```python
from build123d import *

# Parameters (mm, degrees)
F1_DEPTH  = 10
F2_W      = 5
F2_H      = 20
F3_DEPTH  = 20
F5_DEPTH  = 3
F8_DEPTH  = 12
F9_R      = 5.5
F10_DEPTH = 20
F11_R     = 2.65
F12_DEPTH = 25
F13_R     = 3.15
F14_DEPTH = 25
F16_DEPTH = 20
F18_DEPTH = 25


with BuildPart() as f1:
    # F0 (on Front) → F1 (new body, symmetric)
    with BuildSketch(Plane.XZ):
        Polygon((-10, 20), (-10, -20), (10, -10), (10, 10), align=None)
    extrude(amount=F1_DEPTH, both=True)

    # F2 (on face) → F3 (join, through all)
    with BuildSketch(Plane.XZ.offset(10)):
        with Locations((12.5, 0)):
            Rectangle(F2_W, F2_H)
    extrude(amount=-F3_DEPTH)

    # F4 (on face) → F5 (cut)
    with BuildSketch(Plane.YZ.offset(15)):
        Polygon((0, -4.75), (4.113620668, -2.375), (4.113620668, 2.375), (0, 4.75), (-4.1136206679, 2.375), (-4.1136206679, -2.375), align=None)
    extrude(amount=-F5_DEPTH, mode=Mode.SUBTRACT)

    # F7 (on offset) → F8 (cut, through all)
    with BuildSketch(Plane.XZ.offset(6)):
        Polygon((-10, 17), (-10, -17), (10, -7), (10, 7), align=None)
    extrude(amount=-F8_DEPTH, mode=Mode.SUBTRACT)

    # F9 (on face) → F10 (join, through all)
    with BuildSketch(Plane.XZ.offset(10)):
        with Locations((-10, 20)):
            Circle(F9_R)
        with Locations((-10, -20)):
            Circle(F9_R)
    extrude(amount=-F10_DEPTH)

    # F11 (on face) → F12 (cut)
    with BuildSketch(Plane.YZ.offset(12)):
        Circle(F11_R)
    extrude(amount=-F12_DEPTH, mode=Mode.SUBTRACT)

    # F13 (on face) → F14 (cut)
    with BuildSketch(Plane(origin=(0, 10, 0), x_dir=(-1, 0, 0), z_dir=(0, 1, 0))):
        with Locations((10, -20)):
            Circle(F13_R)
        with Locations((10, 20)):
            Circle(F13_R)
    extrude(amount=-F14_DEPTH, mode=Mode.SUBTRACT)

    # F15 (on face) → F16 (join, through all)
    with BuildSketch(Plane(origin=(0, 10, 0), x_dir=(-1, 0, 0), z_dir=(0, 1, 0))):
        Polygon((-10, 10), (5.0806504495, 17.5403252248), (5.0806504495, 22.4596747752), (-15, 10), align=None)
        Polygon((5.0806504495, -22.4596747752), (5.0806504495, -17.5403252248), (-10, -10), (-15, -10), align=None)
    extrude(amount=-F16_DEPTH)

    # F17 (on face) → F18 (cut)
    with BuildSketch(Plane.XZ.offset(10)):
        Polygon((-3.2343349885, 0), (-10, 14.5), (-10, -14.5), align=None)
    extrude(amount=-F18_DEPTH, mode=Mode.SUBTRACT)


solid = f1.part
```
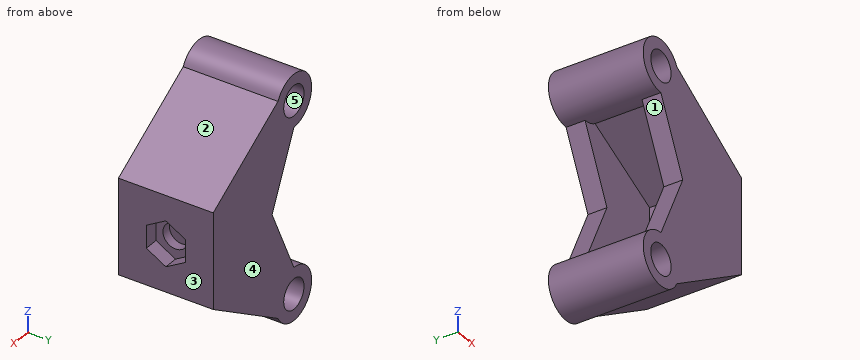
Geometry check sheet. Reference: the model listing, model coordinates, mm. Face numbers are marked on the shaded views. A direction names the side the tool comes from. Give positions to 0.01 mm unless a question says otherwise; leave off trailing zeros. Order: outer loops, then holes, each group sorted by start corner. A loop starts at its lowest first (then second) coordinate and runs counter-clockwise, first axis right, second up.
1. Section check B-B, the plane z = 20. Enter the section's corners in (x, y).
2. Access from +Z, -Z, +X, -X, +Y, -Y to the whole of each face (thin tool, end or side, straight path). Record for the marked faces 1 and 2.
3. Gauge pin test, flat ends, axial feed: pin 1 Ø10 at (y, z) = (-1, -11.5) entering from -X; pin 2 Ø2 at (y, z) = (6, -5.5) entering from -X; pin 3 Ø5 at (x, z) = (12, 17) entering from +Y; pin 4 Ø1 at (y, z) = (-3.5, 15.5) entering from -X. Record the tip position at first contact, or that the pin passes through.
4. Section check A-A, the plane y = 1.5. Enter the section's corners in (x, z), and give its area (3 significant figures).
5. Release check for a two-part mould opening along X. For the marked faces 3, 4 and 5 record: pulls with the +X half, pulls with the -X half, needs draft (parallel to the pull), parting line crosses it, or undercut.
6. Thickness scan on L1, parallel to Z at x = -10, y = 3.75; L2, parallel to Y at x = -7, z = 11.5; L3, parallel to Z at x = -12.5, y = 2. Record the ranges inside material, lowest first.
7. Section check C-C, the plane x = 0.5. Enter the section's corners in (y, z).
8. Section check D-D, the plane y = 7. Enter the section's corners in (x, z), and give its area (3 significant figures).
Values follow:
1. outline: (-15.5, -10) - (-13.15, -10) - (-13.15, 10) - (-15.5, 10) - close; (-6.85, -10) - (-1.12, -10) - (-1.12, 10) - (-6.85, 10) - close
2. face 1: -X, +Y, -Y
2. face 2: +Z, +X, +Y, -Y
3. pin 1: stops at x = -14.24
3. pin 2: stops at x = -6.27
3. pin 3: passes through
3. pin 4: stops at x = -13.77
4. outline: (-6.91, -15.45) arc R5.5 ccw (long way) to (-5.08, -22.46) - (15, -10) - (15, -3.88) - (12, -3.88) - (12, -2.18) - (10, -2.18) - (10, -7) - close; (-6.91, 15.45) - (10, 7) - (10, 2.18) - (12, 2.18) - (12, 3.88) - (15, 3.88) - (15, 10) - (-5.08, 22.46) arc R5.5 ccw (long way) to start; hole circle Ø6.3 at (-10, -20); hole circle Ø6.3 at (-10, 20)
4. area: 424 mm2
5. face 3: pulls with the +X half
5. face 4: needs draft
5. face 5: undercut
6. L1: z = -25.5 to -23.15, -16.85 to -14.5, 14.5 to 16.85, 23.15 to 25.5
6. L2: y = -10 to -6, 6 to 10
6. L3: z = -24.9 to -21.92, -18.08 to -15.1, 15.1 to 18.08, 21.92 to 24.9
7. outline: (-10, -19) - (10, -19) - (10, 19) - (-10, 19) - close; hole (-6, -11.75) - (6, -11.75) - (6, 11.75) - (-6, 11.75) - close
8. outline: (-10, -14.5) arc R5.5 ccw (long way) to (-5.08, -22.46) - (15, -10) - (15, 10) - (-5.08, 22.46) arc R5.5 ccw (long way) to (-10, 14.5) - (-3.23, 0) - close; hole circle Ø6.3 at (-10, -20); hole circle Ø6.3 at (-10, 20)
8. area: 829 mm2
